Build history of the part. All positions in model axes, mm. Face numbers are marked on the shaded views. A direction names the side the tool comes from. Give positions to 0.01 mm unless a question says otherwise; leave off trailing zeros. Order: outer loops, then holes, each group sorted by start corner. A loop starts at its lowest first (then second) coordinate and runs counter-clockwise, first axis right, second up. Notation, with made-up numbers: (-1.5, 42.25) - (57.5, 42.25) arc R24 ccw to (57.5, 81.25) - close; hole circle Ø1 at (77, -3.75). An arc over 180 degrees is marked (long way). One line per item, written item: value.
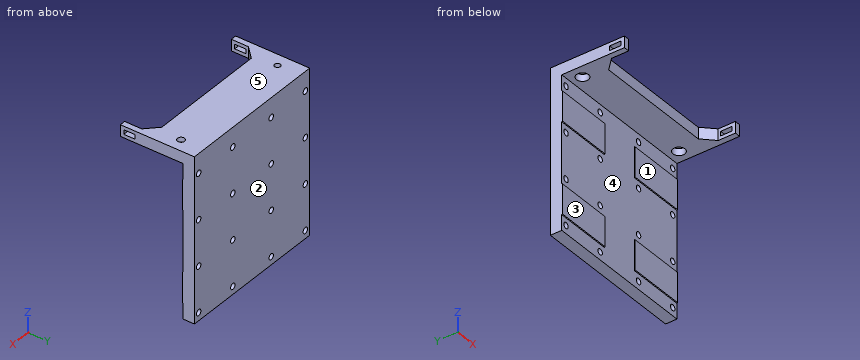
```python
from build123d import *

# Parameters (mm, degrees)
SKETCH1_W               = 135
SKETCH1_H               = 134
BOSS_EXTRUDE1_DEPTH     = 10
SKETCH2_W               = 50
SKETCH2_H               = 27
BOSS_EXTRUDE2_DEPTH     = 0.5
CUT_EXTRUDE1_DEPTH      = 96.630800478
CUT_EXTRUDE1_DEPTH_BACK = 96.630800478
SKETCH3_R               = 2.6
BOSS_EXTRUDE3_START     = 67
SKETCH4_W               = 135
SKETCH4_H               = 40
BOSS_EXTRUDE3_DEPTH     = 10
CUT_EXTRUDE2_DEPTH      = 107.701686959
CUT_EXTRUDE2_DEPTH_BACK = 184.701686959
CUT_EXTRUDE2_START      = 77
SKETCH5_R               = 2.488859202
SKETCH5_R_2             = 3.1003276
CHAMFER1_SIZE           = 0.5
CUT_EXTRUDE3_START      = 67
SKETCH6_R               = 5.25
CUT_EXTRUDE3_DEPTH      = 6
BOSS_EXTRUDE4_START     = -67.5
SKETCH7_W               = 10
SKETCH7_H               = 25.09735907
SKETCH7_W_2             = 4
SKETCH7_H_2             = 10
BOSS_EXTRUDE4_DEPTH     = 5
BOSS_EXTRUDE5_START     = 67.5
SKETCH7_2_W             = 10
SKETCH7_2_H             = 25.09735907
SKETCH7_2_W_2           = 4
SKETCH7_2_H_2           = 10
BOSS_EXTRUDE5_DEPTH     = 5
CHAMFER2_SIZE           = 10


with BuildPart() as part:
    # Sketch1 → Boss-Extrude1 (new body)
    with BuildSketch(Plane(origin=(0, 0, 0), x_dir=(1, 0, 0), z_dir=(0, 1, 0))):
        Rectangle(SKETCH1_W, SKETCH1_H)
    extrude(amount=BOSS_EXTRUDE1_DEPTH)

    # Sketch2 → Boss-Extrude2 (add)
    with BuildSketch(Plane(origin=(0, 0, 0), x_dir=(1, 0, 0), z_dir=(0, 1, 0))):
        with Locations((-42.5, 40)):
            Rectangle(SKETCH2_W, SKETCH2_H)
        with Locations((-42.5, -40)):
            Rectangle(SKETCH2_W, SKETCH2_H)
        with Locations((42.5, -40)):
            Rectangle(SKETCH2_W, SKETCH2_H)
        with Locations((42.5, 40)):
            Rectangle(SKETCH2_W, SKETCH2_H)
    extrude(amount=-BOSS_EXTRUDE2_DEPTH)

    # Sketch3 → Cut-Extrude1 (cut, two sides: drawn at the far end of the back side and taken through both)
    with BuildSketch(Plane(origin=(0, 0, 0), x_dir=(1, 0, 0), z_dir=(0, 1, 0)).offset(-CUT_EXTRUDE1_DEPTH_BACK)):
        with Locations(Location((-62.5, 20, 0), (0, 0, 270))):
            Circle(SKETCH3_R)
        with Locations(Location((-22.5, 20, 0), (0, 0, 270))):
            Circle(SKETCH3_R)
        with Locations(Location((-22.5, 60, 0), (0, 0, 270))):
            Circle(SKETCH3_R)
        with Locations(Location((-62.5, 60, 0), (0, 0, 270))):
            Circle(SKETCH3_R)
        with Locations(Location((-62.5, -60, 0), (0, 0, 90))):
            Circle(SKETCH3_R)
        with Locations(Location((-22.5, -60, 0), (0, 0, 90))):
            Circle(SKETCH3_R)
        with Locations(Location((-22.5, -20, 0), (0, 0, 90))):
            Circle(SKETCH3_R)
        with Locations(Location((-62.5, -20, 0), (0, 0, 90))):
            Circle(SKETCH3_R)
        with Locations(Location((62.5, -20, 0), (0, 0, 270))):
            Circle(SKETCH3_R)
        with Locations(Location((22.5, -20, 0), (0, 0, 270))):
            Circle(SKETCH3_R)
        with Locations(Location((22.5, -60, 0), (0, 0, 270))):
            Circle(SKETCH3_R)
        with Locations(Location((62.5, -60, 0), (0, 0, 270))):
            Circle(SKETCH3_R)
        with Locations(Location((62.5, 60, 0), (0, 0, 90))):
            Circle(SKETCH3_R)
        with Locations(Location((22.5, 60, 0), (0, 0, 90))):
            Circle(SKETCH3_R)
        with Locations(Location((22.5, 20, 0), (0, 0, 90))):
            Circle(SKETCH3_R)
        with Locations(Location((62.5, 20, 0), (0, 0, 90))):
            Circle(SKETCH3_R)
    extrude(amount=CUT_EXTRUDE1_DEPTH + CUT_EXTRUDE1_DEPTH_BACK, mode=Mode.SUBTRACT)

    # Sketch4 → Boss-Extrude3 (add)
    with BuildSketch(Plane.XY.offset(BOSS_EXTRUDE3_START)):
        with Locations((0, -10)):
            Rectangle(SKETCH4_W, SKETCH4_H)
    extrude(amount=BOSS_EXTRUDE3_DEPTH)

    # Sketch5 → Cut-Extrude2 (cut, two sides: drawn at the far end of the back side and taken through both)
    with BuildSketch(Plane.XY.offset(CUT_EXTRUDE2_START - CUT_EXTRUDE2_DEPTH_BACK)):
        with Locations((-56.5, -10)):
            Circle(SKETCH5_R)
        with Locations((56.5, -10)):
            Circle(SKETCH5_R_2)
    extrude(amount=CUT_EXTRUDE2_DEPTH + CUT_EXTRUDE2_DEPTH_BACK, mode=Mode.SUBTRACT)

    # Chamfer1
    chamfer1_edges = [part.edges().sort_by_distance(p)[0] for p in [
        (42.5, -0.5, 26.5),
        (42.5, -0.5, 53.5),
        (-42.5, -0.5, 53.5),
        (-42.5, -0.5, 26.5),
        (-42.5, -0.5, -53.5),
        (-42.5, -0.5, -26.5),
        (42.5, -0.5, -26.5),
        (42.5, -0.5, -53.5),
    ]]
    chamfer(chamfer1_edges, length=CHAMFER1_SIZE - 0.0001)  # a hair under: the kernel refuses the full size

    # Sketch6 → Cut-Extrude3 (cut)
    with BuildSketch(Plane.XY.offset(CUT_EXTRUDE3_START)):
        with Locations((56.5, -10)):
            Circle(SKETCH6_R)
        with Locations((-56.5, -10)):
            Circle(SKETCH6_R)
    extrude(amount=CUT_EXTRUDE3_DEPTH, mode=Mode.SUBTRACT)

    # Sketch7 → Boss-Extrude4 (add)
    with BuildSketch(Plane(origin=(0, 0, 0), x_dir=(0, 0, -1), z_dir=(1, 0, 0)).offset(BOSS_EXTRUDE4_START)):
        with Locations((-72, -42.548679535)):
            Rectangle(SKETCH7_W, SKETCH7_H)
        with Locations((-72, -47.09735907)):
            Rectangle(SKETCH7_W_2, SKETCH7_H_2, mode=Mode.SUBTRACT)
    extrude(amount=BOSS_EXTRUDE4_DEPTH)

    # Sketch7<2> → Boss-Extrude5 (add)
    with BuildSketch(Plane(origin=(0, 0, 0), x_dir=(0, 0, -1), z_dir=(1, 0, 0)).offset(BOSS_EXTRUDE5_START)):
        with Locations((-72, -42.548679535)):
            Rectangle(SKETCH7_2_W, SKETCH7_2_H)
        with Locations((-72, -47.09735907)):
            Rectangle(SKETCH7_2_W_2, SKETCH7_2_H_2, mode=Mode.SUBTRACT)
    extrude(amount=-BOSS_EXTRUDE5_DEPTH)

    # Chamfer2
    chamfer2_edges = [part.edges().sort_by_distance(p)[0] for p in [
        (-62.5, -30, 72),
        (62.5, -30, 72),
    ]]
    chamfer(chamfer2_edges, length=CHAMFER2_SIZE)


solid = part.part
```
(1) Slice it at A-A, the plane y = -10. Give the cut face in (x, z), and give its area (3 significant figures).
Completed:
outline: (-67.5, 67) - (-61.75, 67) - (-61.75, 73) - (-58.99, 73) - (-58.99, 77) - (-67.5, 77) - close; (-54.01, 73) - (-51.25, 73) - (-51.25, 67) - (51.25, 67) - (51.25, 73) - (53.4, 73) - (53.4, 77) - (-54.01, 77) - close; (59.6, 73) - (61.75, 73) - (61.75, 67) - (67.5, 67) - (67.5, 77) - (59.6, 77) - close
area: 1,180 mm²
(2) Slice it at C-C, the plane x = 22.5. Count the separate pieces of the cut face and the enclosed holes in it, and give its area (3 significant figures).
Completed:
separate pieces: 5
enclosed holes: 0
area: 1,560 mm²
(3) 3-axis set-ups, long thin cutter, end or side, ignore diameter. For the marked faces 1 and 2: which of +Z, -Z, +X, -X, +Y, -Y reach the whole face in a straight line?
Completed:
face 1: -Z, +X, -X, -Y
face 2: +Z, -Z, +X, -X, +Y
(4) Drill centre lines: line 1 (X direction, y = -10, z = 74.6); line 2 (X direction, y = 6, z = 60); line 3 (X direction, y = 6.5, z = -18). Where is each one in solid material? Low to high.
Completed:
line 1: -67.5 to -58.99, -54.01 to 53.4, 59.6 to 67.5
line 2: -67.5 to -65.1, -59.9 to -25.1, -19.9 to 19.9, 25.1 to 59.9, 65.1 to 67.5
line 3: -67.5 to -64.16, -60.84 to -24.16, -20.84 to 20.84, 24.16 to 60.84, 64.16 to 67.5
(5) Pin check, flat tips, straight feed: P1, Ø8.5, axis at x = -22.5, z = -60, coming from the -Y side; P2, Ø2, axis at x = 46.5, y = -20.5, coming from the -Z side; P3, Ø6, axis at x = 33, z = -33, coming from the -Y side; P4, Ø3, axis at x = -62.5, z = -20, coming from the +Y side. Stop position of each tip, or through.
Completed:
P1: y = 0
P2: z = 67
P3: y = -0.5
P4: through
(6) Pull direction Z, two halves, no side cores. Call the marked faces 3, 4 and 5: +Z half, -Z half, draft (parallel to the pull), parting line (faces both ways), or undercut.
Completed:
face 3: draft
face 4: undercut
face 5: +Z half
(7) Slice it at B-B, the plane z = 60. Give the cut face in (x, y), and give its area (3 significant figures).
Completed:
outline: (-67.5, 0) - (-65.1, 0) - (-65.1, 10) - (-67.5, 10) - close; (-59.9, 0) - (-25.1, 0) - (-25.1, 10) - (-59.9, 10) - close; (-19.9, 0) - (19.9, 0) - (19.9, 10) - (-19.9, 10) - close; (25.1, 0) - (59.9, 0) - (59.9, 10) - (25.1, 10) - close; (65.1, 0) - (67.5, 0) - (67.5, 10) - (65.1, 10) - close
area: 1,140 mm²
